Geometry: see drawing. Coordinates: mm, zero at the bounding-box minimum. A direction names the side the tool comes from. Give positions to 0.01 mm unless a question says otherwise; leave off trailing zeros. Loops run counter-clockwise (first coordinate to the right, second up) from the corner with the lowest first, then second, coordinate; pieces in that order, holes last. Notation, with made-up numbers: M 30.5,55.5 L 76.5,55.5 A14 cw 76.5,59.5 Z; hole C 14,26 d3. An arc over 180 degrees is marked long. Answer in a Markdown table with one row per item.
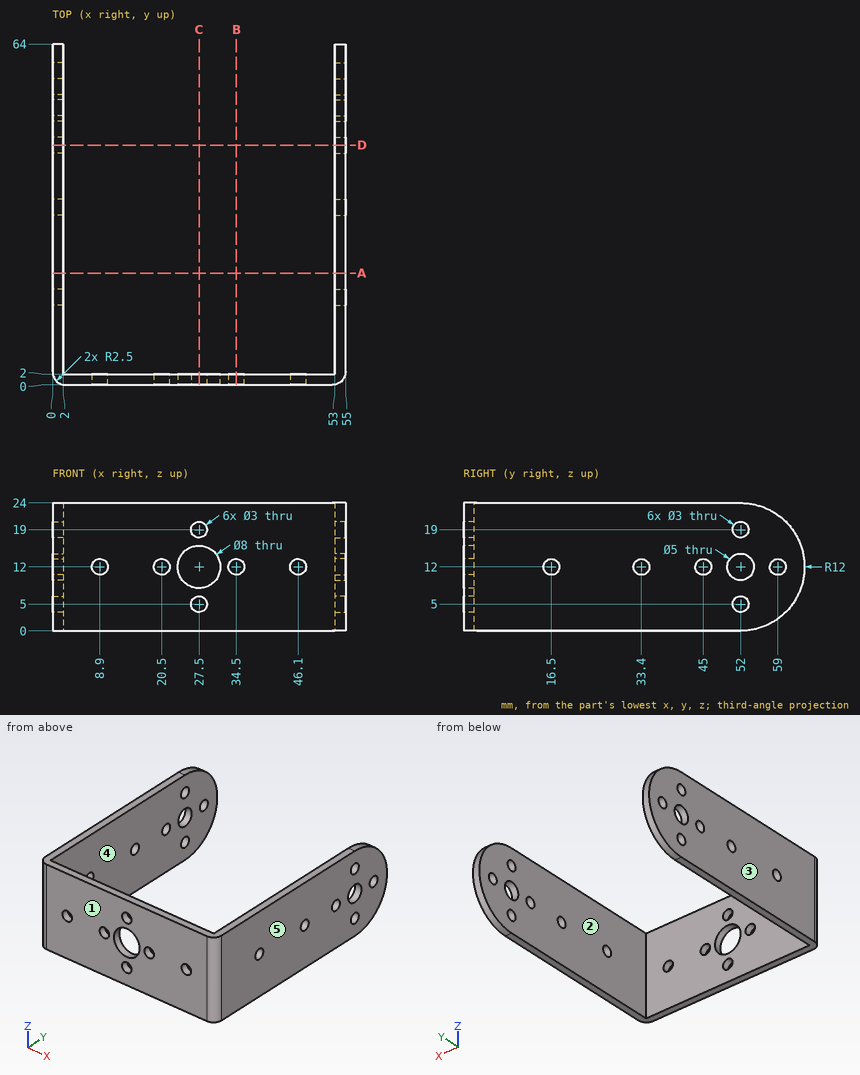
1) Set-up query: the marked faces 1 and 2. Return all of +Z, -Z, +X, -X, +Y, -Y with unobstructed straight access to the full face (end or side cutting, diameter ignored); none if empty.
Reply:
| item | result |
|---|---|
| face 1 | +Z, -Z, +X, -X, -Y |
| face 2 | +Z, -Z, +Y |
2) Section B-B, the plane x = 34.5. Return loops of the section in (y, z).
Reply:
| item | result |
|---|---|
| outline | M 0,0 L 2,0 L 2,10.5 L 0,10.5 Z; M 0,13.5 L 2,13.5 L 2,24 L 0,24 Z |
3) Section D-D, the plane y = 45. Return loops of the section in (x, z).
Reply:
| item | result |
|---|---|
| outline | M 0,0 L 2,0 L 2,10.5 L 0,10.5 Z; M 0,13.5 L 2,13.5 L 2,24 L 0,24 Z; M 53,0 L 55,0 L 55,10.5 L 53,10.5 Z; M 53,13.5 L 55,13.5 L 55,24 L 53,24 Z |
4) Material intervals for L1, parallel to X at y = 28, z = 21; L2, parallel to Y at x = 0.95, z = 12; L3, parallel to Y at x = 0.6, z = 12, sorted ascending.
Reply:
| item | result |
|---|---|
| L1 | x = 0 to 2, 53 to 55 |
| L2 | y = 0.54 to 15, 18 to 31.9, 34.9 to 43.5, 46.5 to 49.5, 54.5 to 57.5, 60.5 to 64 |
| L3 | y = 0.88 to 15, 18 to 31.9, 34.9 to 43.5, 46.5 to 49.5, 54.5 to 57.5, 60.5 to 64 |
5) Section A-A, the plane y = 21. Return loops of the section in (x, z), then the cut area to 3 significant figures.
Reply:
| item | result |
|---|---|
| outline | M 0,0 L 2,0 L 2,24 L 0,24 Z; M 53,0 L 55,0 L 55,24 L 53,24 Z |
| area | 96.0 mm² |
6) Pull-direction query (X, two-part tool) for the marked faces 3, 4 and 5; classes: released by +X, released by -X, zero draft, split by the parting line, or undercut.
Reply:
| item | result |
|---|---|
| face 3 | released by -X |
| face 4 | undercut |
| face 5 | released by +X |
7) Pin query (flat end, axial travel): pin 1 Ø2.5 at (y, z) = (59, 12) entering from -X; pin 2 Ø2 at (y, z) = (43, 6) entering from -X; pin 3 Ø4 at (x, z) = (46.1, 12) entering from +Y. Return the tip coordinate at first contact, or that it passes through.
Reply:
| item | result |
|---|---|
| pin 1 | passes through |
| pin 2 | stops at x = 0 |
| pin 3 | stops at y = 2 |
8) Section C-C, the plane x = 27.5. Return loops of the section in (y, z), then the cut area to 3 significant figures.
Reply:
| item | result |
|---|---|
| outline | M 0,0 L 2,0 L 2,3.5 L 0,3.5 Z; M 0,6.5 L 2,6.5 L 2,8 L 0,8 Z; M 0,16 L 2,16 L 2,17.5 L 0,17.5 Z; M 0,20.5 L 2,20.5 L 2,24 L 0,24 Z |
| area | 20.0 mm² |
